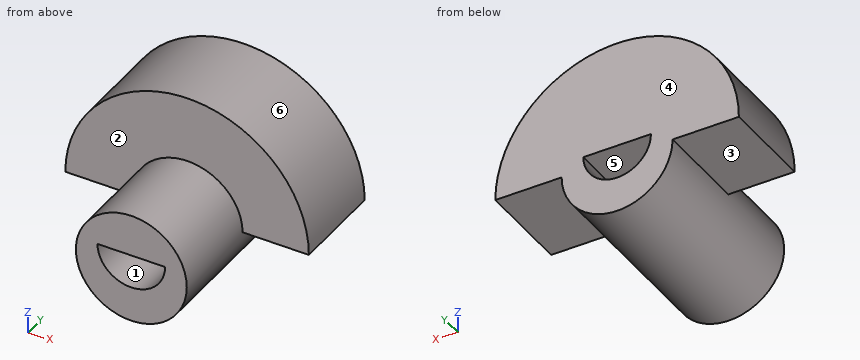
from build123d import *

# Parameters (mm, degrees)
BOSS_EXTRUDE1_DEPTH = 7
SKETCH2_R           = 4.1
BOSS_EXTRUDE2_DEPTH = 7
CUT_EXTRUDE1_DEPTH  = 15


with BuildPart() as part:
    # Sketch1 → Boss-Extrude1 (new body)
    with BuildSketch(Plane(origin=(0, 0, 0), x_dir=(1, 0, 0), z_dir=(0, 1, 0))):
        with BuildLine():
            Line((4.1, 0), (9, 0))
            ThreePointArc((9, 0), (0, -9), (-9, 0))
            Line((-9, 0), (-4.1, 0))
            ThreePointArc((-4.1, 0), (0, 4.1), (4.1, 0))
        make_face()
    extrude(amount=BOSS_EXTRUDE1_DEPTH)

    # Sketch2 → Boss-Extrude2 (add)
    with BuildSketch(Plane.XZ):
        Circle(SKETCH2_R)
    extrude(amount=BOSS_EXTRUDE2_DEPTH)

    # Sketch3 → Cut-Extrude1 (cut, through all)
    with BuildSketch(Plane(origin=(0, 7, 0), x_dir=(1, 0, 0), z_dir=(0, 1, 0))):
        with BuildLine():
            Line((2.5, -1), (-2.5, -1))
            ThreePointArc((-2.5, -1), (0, 1.5), (2.5, -1))
        make_face()
    extrude(amount=-CUT_EXTRUDE1_DEPTH, mode=Mode.SUBTRACT)


solid = part.part
Check sheet for the modelled part. Datum: model origin and axes. Units: mm. Face numbers are marked on the shaded views. A direction names the side the tool comes from. Coordinates: 2 decimals unless noted, no trailing zeros. Write each loop counter-clockwise with the first axis right and the second up, starting at its lowest first coordinate (ties: lowest second). Pieces come first, ordered by that corner, then holes. Notation, with made-up numbers: M -31.75,21.5 L 3.25,21.5 A22 ccw 3.25,29.5 Z; hole C 47,-10.5 d10. An arc over 180 degrees is marked long. Answer as CSV lines item,"result".
Q1. Cross-section at A-A (x = -1.5). Record the boundary of the cut face in (y, z).
Check result:
outline,"M -7,-3.82 L 7,-3.82 L 7,-1 L -7,-1 Z; M -7,1 L 7,1 L 7,8.87 L 0,8.87 L 0,3.82 L -7,3.82 Z"
Q2. Cross-section at B-B (y = -3.25). Record the boundary of the cut face in (x, z).
Check result:
outline,"C 0,0 d8.2; hole M -2.5,1 A2.5 ccw 2.5,1 Z"
Q3. Cross-section at D-D (x = 0.5). Record the boundary of the cut face in (y, z).
Check result:
outline,"M -7,-4.07 L 7,-4.07 L 7,-1.45 L -7,-1.45 Z; M -7,1 L 7,1 L 7,8.99 L 0,8.99 L 0,4.07 L -7,4.07 Z"
Q4. Material ranges on probe 1 along Y at (x, z) = (6.75, 5); probe 2 along X at (y, z) = (-3.5, -0.75); probe 3 along X at (y, z) = (-4.5, 0.5), recorded low to high. Write a range as from..to.
Check result:
probe 1,"0..7"
probe 2,"-4.03..-1.79, 1.79..4.03"
probe 3,"-4.07..-2.45, 2.45..4.07"
Q5. Set-up check for the marked faces 1, 2 and 3: record each of +Z, -Z, +X, -X, +Y, -Y from which the full face is reachable in a straight line by a thin tool's end or side.
Check result:
face 1,"+Y, -Y"
face 2,"+Z, -Y"
face 3,"-Z, -X, +Y, -Y"
Q6. Mould release check, pull along Z, two halves, no side actions. Record for the marked faces 4, 5 and 6: released by +Z, released by -Z, zero draft, split by the parting line, or undercut.
Check result:
face 4,"zero draft"
face 5,"undercut"
face 6,"released by +Z"
Q7. Cross-section at C-C (z = 3). Record the boundary of the cut face in (x, y).
Check result:
outline,"M -8.49,0 L -2.79,0 L -2.79,-7 L 2.79,-7 L 2.79,0 L 8.49,0 L 8.49,7 L -8.49,7 Z"
Q8. Go/stop test with flat-tipped pins: pin 1 (3 mm diameter, centred on x = -6, y = 0.5, fed in from +Z); pin 2 (5.5 mm diameter, centred on x = 7.5, y = 2.5, fed in from -Z); pin 3 (1 mm diameter, centred on x = -4.5, z = 7.5, fed in from -Y). Record where each tip stops, or that it passes through.
Check result:
pin 1,"z = 7.79"
pin 2,"z = 0"
pin 3,"y = 0"
